```python
from build123d import *

# Parameters (mm, degrees)
SKETCH_1_R                     = 25
SKETCH_1_R_2                   = 15
EXTRUDE_1_DEPTH                = 22.5
SKETCH_2_W                     = 92
SKETCH_2_H                     = 14
EXTRUDE_2_DEPTH                = 62
EXTRUDE_3_DEPTH                = 6
RIB_1_REACH                    = 123.639
SKETCH_4_WALL_W                = 303.26037525
SKETCH_4_WALL_H                = 12
FILLET_1_R                     = 8
HOLE_WIZARD_M1_6_1_D           = 8
HOLE_WIZARD_M1_6_1_CBORE_D     = 12
HOLE_WIZARD_M1_6_1_CBORE_DEPTH = 2
HOLE_WIZARD_M6_1_D             = 5
HOLE_WIZARD_M8_1_D             = 6.8
PATTERN_CIRCULAR_1_COUNT       = 6
HOLE_WIZARD_M4_2_D             = 3.3
HOLE_WIZARD_M4_2_DEPTH         = 11.5
HOLE_WIZARD_M4_2_TIP           = 0.991420021


with BuildPart() as part:
    # Sketch 1 → Extrude 1 (new, symmetric)
    with BuildSketch(Plane.XY):
        with Locations(Location((0, 0, 0), (0, 0, 180))):
            Circle(SKETCH_1_R)
        with Locations(Location((0, 0, 0), (0, 0, 180))):
            Circle(SKETCH_1_R_2, mode=Mode.SUBTRACT)
    extrude(amount=EXTRUDE_1_DEPTH, both=True)



with BuildPart() as body_2:
    # Sketch 2 → Extrude 2 (new, symmetric)
    with BuildSketch(Plane.XY):
        with Locations((0, -87)):
            Rectangle(SKETCH_2_W, SKETCH_2_H)
    extrude(amount=EXTRUDE_2_DEPTH, both=True)


with BuildPart() as part_1:
    add(part.part)

    add(body_2.part)  # Extrude 3 merges body 2
    # Sketch 3 → Extrude 3 (add, symmetric)
    with BuildSketch(Plane.XY):
        with BuildLine():
            Line((-24.238210613, 6.124471102), (-46, -80))
            Line((-46, -80), (46, -80))
            Line((46, -80), (24.238210613, 6.124471102))
            ThreePointArc((24.238210613, 6.124471102), (0, -25), (-24.238210613, 6.124471102))
        make_face()
    extrude(amount=EXTRUDE_3_DEPTH, both=True)

    # Sketch 4 wall → Rib 1 (add, up to next)
    with BuildSketch(Plane(origin=(0, -59.5, 26.5), x_dir=(0, -0.707106781187, 0.707106781187), z_dir=(0, -0.707106781187, -0.707106781187)), mode=Mode.PRIVATE) as rib_1_sk1:
        Rectangle(SKETCH_4_WALL_W, SKETCH_4_WALL_H)
    rib_1_tool1 = extrude(rib_1_sk1.sketch, amount=RIB_1_REACH, mode=Mode.PRIVATE) - part_1.part
    rib_1 = rib_1_tool1.solids().sort_by_distance((0, -59.5, 26.5))[0]
    add(rib_1)

    # Mirror 1: Rib 1 across plane
    add(rib_1.mirror(Plane.XY))

    # Fillet 1
    fillet_1_edges = [part_1.edges().sort_by_distance(p)[0] for p in [
        (-46, -87, -62),
        (46, -87, -62),
        (-46, -87, 62),
        (46, -87, 62),
    ]]
    fillet(fillet_1_edges, radius=FILLET_1_R)

    # Hole Wizard M1.6 _ _ _ _ _1 (through all)
    with Locations(Plane(origin=(-38, -80, 54), x_dir=(0, 0, 1), z_dir=(0, 1, 0))):
        with Locations((0, 0), (0, 76), (-108, 76), (-108, 0)):
            CounterBoreHole(HOLE_WIZARD_M1_6_1_D / 2, HOLE_WIZARD_M1_6_1_CBORE_D / 2, HOLE_WIZARD_M1_6_1_CBORE_DEPTH)

    # Hole Wizard M6 _ _1 (through all)
    with Locations(Plane(origin=(-22.914678554, -34.420983867, 6), x_dir=(1, 0, 0), z_dir=(0, 0, 1))):
        with Locations((0, 0)):
            Hole(HOLE_WIZARD_M6_1_D / 2)

    # Hole Wizard M8 _ _1 (through all)
    with Locations(Plane(origin=(24.290456281, -37.484031993, 6), x_dir=(1, 0, 0), z_dir=(0, 0, 1))):
        with Locations((0, 0)):
            Hole(HOLE_WIZARD_M8_1_D / 2)

    # Sketch 11 → Hole Wizard M1.6 _ _ _ _ _2 (revolve, cut)
    with BuildSketch(Plane(origin=(-0.334351045, -80, -52.911409403), x_dir=(0, 0, 1), z_dir=(1, 0, 0))):
        Polygon((0, 0), (0, 14), (4, 14), (4, 2), (6, 2), (6, 0), align=None)
    revolve(axis=Axis((-0.334351045, -73.65, -52.911409403), (0, -1, 0)), mode=Mode.SUBTRACT)

    # Sketch 15 → Hole Wizard M4 _ _1 (revolve, cut)
    with BuildSketch(Plane(origin=(0, 20, 22.5), x_dir=(0, -1, 0), z_dir=(1, 0, 0))):
        Polygon((0, 0), (0, 12.491420021), (1.65, 11.5), (1.65, 0), align=None)
    hole_wizard_m4_1 = revolve(axis=Axis((0, 20, 28.85), (0, 0, -1)), mode=Mode.SUBTRACT)

    # Pattern Circular 1: Hole Wizard M4 _ _1 ×6 about axis
    pattern_circular_1_axis = Axis((0, 0, 0), (0, 0, 1))
    for i in range(1, PATTERN_CIRCULAR_1_COUNT):
        add(hole_wizard_m4_1.rotate(pattern_circular_1_axis, i * 360 / PATTERN_CIRCULAR_1_COUNT), mode=Mode.SUBTRACT)

    # Mirror 2: Hole Wizard M4 _ _1 across plane
    add(hole_wizard_m4_1.mirror(Plane.XY), mode=Mode.SUBTRACT)

    # Mirror 2 copy 1 sketch → Mirror 2 copy 1 (revolve, cut)
    with BuildSketch(Plane(origin=(-17.320508076, 10, -22.5), x_dir=(0.8660254037844386, -0.5000000000000001, 0), z_dir=(0.5000000000000001, 0.8660254037844386, 0))):
        Polygon((0, 0), (0, -12.491420021), (1.65, -11.5), (1.65, 0), align=None)
    revolve(axis=Axis((-17.320508076, 10, -28.85), (0, 0, -1)), mode=Mode.SUBTRACT)

    # Mirror 2 copy 2 sketch → Mirror 2 copy 2 (revolve, cut)
    with BuildSketch(Plane(origin=(-17.320508076, -10, -22.5), x_dir=(0.8660254037844387, 0.4999999999999998, 0), z_dir=(-0.4999999999999998, 0.8660254037844387, 0))):
        Polygon((0, 0), (0, -12.491420021), (1.65, -11.5), (1.65, 0), align=None)
    revolve(axis=Axis((-17.320508076, -10, -28.85), (0, 0, -1)), mode=Mode.SUBTRACT)

    # Mirror 2 copy 3 sketch → Mirror 2 copy 3 (revolve, cut)
    with BuildSketch(Plane(origin=(0, -20, -22.5), x_dir=(0, 1, 0), z_dir=(-1, 0, 0))):
        Polygon((0, 0), (0, -12.491420021), (1.65, -11.5), (1.65, 0), align=None)
    revolve(axis=Axis((0, -20, -28.85), (0, 0, -1)), mode=Mode.SUBTRACT)

    # Mirror 2 copy 4 sketch → Mirror 2 copy 4 (revolve, cut)
    with BuildSketch(Plane(origin=(17.320508076, -10, -22.5), x_dir=(-0.8660254037844384, 0.5000000000000004, 0), z_dir=(-0.5000000000000004, -0.8660254037844384, 0))):
        Polygon((0, 0), (0, -12.491420021), (1.65, -11.5), (1.65, 0), align=None)
    revolve(axis=Axis((17.320508076, -10, -28.85), (0, 0, -1)), mode=Mode.SUBTRACT)

    # Mirror 2 copy 5 sketch → Mirror 2 copy 5 (revolve, cut)
    with BuildSketch(Plane(origin=(17.320508076, 10, -22.5), x_dir=(-0.8660254037844386, -0.5000000000000001, 0), z_dir=(0.5000000000000001, -0.8660254037844386, 0))):
        Polygon((0, 0), (0, -12.491420021), (1.65, -11.5), (1.65, 0), align=None)
    revolve(axis=Axis((17.320508076, 10, -28.85), (0, 0, -1)), mode=Mode.SUBTRACT)

    # Hole Wizard M4 _ _2
    with Locations(Plane(origin=(44.040169247, -72.243772604, 0), x_dir=(-0.244978844097, 0.969528424516, 0), z_dir=(0.969528424516, 0.244978844097, 0))):
        with Locations((0, 0)):
            Hole(HOLE_WIZARD_M4_2_D / 2, depth=HOLE_WIZARD_M4_2_DEPTH)
            with Locations((0, 0, -(HOLE_WIZARD_M4_2_DEPTH + HOLE_WIZARD_M4_2_TIP / 2))):  # 118° drill point
                Cone(0, HOLE_WIZARD_M4_2_D / 2, HOLE_WIZARD_M4_2_TIP, mode=Mode.SUBTRACT)


solid = part_1.part
```
Can you work these out from the model? Positions are in its coordinate system, mm. A direction names the side the tool comes from. Coordinates: 2 decimals unless noted, no trailing zeros. Loops run counter-clockwise (first coordinate to the right, second up) from the corner with the lowest first, then second, coordinate; pieces in that order, holes last. Notation, with made-up numbers: M -17,41.25 L 3,41.25 A10 ccw 3,60.25 Z; hole C -23.5,79.25 d1. An arc over 180 degrees is marked long. Put each result on its own line as item: value. Start each with the question number.
(1) Imagine slicing it at B-B on y = -61. List the corners of the cut face in (x, z) for me, and give its area (3 significant figures).
(2) We'd pull the mould along Z, two halves only. Please class faces 1 (the face through (-0.07, 21.65, -16.83)), 2 (the face through (-17.41, -10.27, 10.18)), 3 (the face through (-41.65, -80.99, 49.24)): +Z half, -Z half, draft (parallel to the pull), parting line (faces both ways), or undercut.
(3) Imagine slicing it at D-D on y = 0. List the corners of the cut face in (x, z) for me.
(4) Will these pins go through, and if not, where does the flat tip stop? pin 1 Ø12 at (x, y) = (20, -32) entering from +Z; pin 2 Ø3 at (x, y) = (17.32, -10) entering from +Z; pin 3 Ø4.5 at (x, y) = (-17.32, -10) entering from +Z; pin 4 Ø3 at (y, z) = (-49.5, -19.5) entering from +X.
(5) Imagine slicing it at A-A on z = -37. List the corners of the cut face in (x, y) for me, and give its area (3 significant figures).
(6) Imagine slicing it at C-C on x = -9.5. List the corners of the cut face in (y, z) for me.
(7) I need wall thicknesses on probe 1 along X at (y, z) = (-88, 54); probe 2 along X at (y, z) = (20, 14); probe 3 along X at (y, z) = (11, -19.5). Which ranges of each line are inside material? Lowest first, please.
(8) Which directions (+Z, -Z, +X, -X, +Y, -Y) give clear straight access to the entire face, cutting with the end or side of a thin tool? Please do faces 4 (the face through (-6, -67, 18)), 5 (the face through (6, -67, 18)), 6 (the face through (-6, -67, -18)), 7 (the face through (-11, -80, -34)).
Worked answers:
1. outline: M -41.2,-6 L -6,-6 L -6,-28 L 6,-28 L 6,-6 L 41.2,-6 L 41.2,6 L 6,6 L 6,28 L -6,28 L -6,6 L -41.2,6 Z
1. area: 1,520 mm2
2. face 1: draft
2. face 2: +Z half
2. face 3: undercut
3. outline: M -25.79,-6 L -25,-6 L -25,-22.5 L -15,-22.5 L -15,22.5 L -25,22.5 L -25,6 L -25.79,6 Z; M 15,-22.5 L 25,-22.5 L 25,-6 L 25.79,-6 L 25.79,6 L 25,6 L 25,22.5 L 15,22.5 Z
4. pin 1: stops at z = 6
4. pin 2: stops at z = 10.91
4. pin 3: stops at z = 22.5
4. pin 4: passes through
5. outline: M -46,-94 L 46,-94 L 46,-80 L 6,-80 L 6,-70 L -6,-70 L -6,-80 L -46,-80 Z
5. area: 1,410 mm2
6. outline: M -94,-62 L -80,-62 L -80,-6 L -23.12,-6 L -23.12,-22.5 L -11.61,-22.5 L -11.61,22.5 L -23.12,22.5 L -23.12,6 L -80,6 L -80,62 L -94,62 Z; M 11.61,-22.5 L 23.12,-22.5 L 23.12,22.5 L 11.61,22.5 Z
7. probe 1: x = -46 to -42, -34 to 34, 42 to 46
7. probe 2: x = -15 to -1.65, 1.65 to 15
7. probe 3: x = -22.45 to -18.63, -16.01 to -10.2, 10.2 to 16.01, 18.63 to 22.45
8. face 4: +Z, -X
8. face 5: +Z, +X
8. face 6: -Z, -X
8. face 7: -Z
